```python
from build123d import *

# Parameters (mm, degrees)
F0_W     = 101.6
F0_H     = 9.525
F0_R     = 1.35255
F0_R_2   = 3.175
F1_DEPTH = 1.70942
F2_R     = 0.762
F3_SIZE  = 1.5875


with BuildPart() as f1:
    # F0 (on Top) → F1 (new body)
    with BuildSketch(Plane.XY):
        with Locations((-50.8, -4.7625)):
            Rectangle(F0_W, F0_H)
        with Locations((-97.63125, -3.96875)):
            Circle(F0_R, mode=Mode.SUBTRACT)
        with Locations((-65.057693, -3.96875)):
            Circle(F0_R, mode=Mode.SUBTRACT)
        with Locations((-50.8, -3.96875)):
            Circle(F0_R_2, mode=Mode.SUBTRACT)
        with Locations((-36.542307, -3.96875)):
            Circle(F0_R, mode=Mode.SUBTRACT)
        with Locations((-3.96875, -3.96875)):
            Circle(F0_R, mode=Mode.SUBTRACT)
    extrude(amount=F1_DEPTH)

    # F2
    f2_edges = [f1.edges().sort_by_distance(p)[0] for p in [
        (-101.6, 0, 0.85471),
        (0, 0, 0.85471),
    ]]
    fillet(f2_edges, radius=F2_R)

    # F3
    f3_edges = [f1.edges().sort_by_distance(p)[0] for p in [
        (0, -9.525, 0.85471),
        (-101.6, -9.525, 0.85471),
    ]]
    chamfer(f3_edges, length=F3_SIZE)


solid = f1.part
```
The listing builds one solid part. Answer for the finished solid, in the listing's coordinates (mm). Coordinates: 2 decimals unless noted, no trailing zeros. Loops run counter-clockwise (first coordinate to the right, second up) from the corner with the lowest first, then second, coordinate; pieces in that order, holes last. Notation, with made-up numbers: M -24,-21 L -1,-21 A7 ccw -1,-11 Z; hole C 63.25,50.25 d8. An arc over 180 degrees is marked long. Answer as CSV lines item,"result". Start each with the question number.
(1) Find the intervals of material crossed by L1, parallel to Y at x = -50.8, z = 1.3 (3 decimals); L2, parallel to X at y = -3.5, z = 0.5; L3, parallel to X at y = -3.25, z = 1.15, in increasing order. Write a range as [from, to].
(2) The part is cut by section A-A (x = -50.8). Give the vertices of the cut face in (y, z) (3 decimals), and give its area (3 significant figures).
(3) The part is cut by section B-B (z = 1.2). State how many separate pieces and enclosed holes the cut face has, and give its area (3 significant figures).
(4) The mould has two halves that part along X. Classify faces 1 (the flat face through (-101.6, -4, 1)), 2 (the flat face through (-51, -9.525, 1)), 3 (the cylindrical face through (-4.26, -5.29, 0.84)): pulls with the +X half, pulls with the -X half, needs draft (parallel to the pull), parting line crosses it, or undercut.
(5) Given pin 1 (2 mm diameter, centred on x = -97.63, y = -3.97, fed in from -Z), flat-ended and moving along its own axis, determine where the tip first touches the part or whether it passes through.
Determined:
1,L1,"[-9.525, -7.144], [-0.794, 0]"
1,L2,"[-101.6, -98.9], [-96.36, -66.33], [-63.79, -53.94], [-47.66, -37.81], [-35.27, -5.24], [-2.7, 0]"
1,L3,"[-101.6, -98.78], [-96.49, -66.2], [-63.91, -53.89], [-47.71, -37.69], [-35.4, -5.11], [-2.82, 0]"
2,outline,"M -9.525,0 L -7.144,0 L -7.144,1.709 L -9.525,1.709 Z; M -0.794,0 L 0,0 L 0,1.709 L -0.794,1.709 Z"
2,area,"5.43 mm2"
3,separate pieces,"1"
3,enclosed holes,"5"
3,area,"910 mm2"
4,face 1,"pulls with the -X half"
4,face 2,"needs draft"
4,face 3,"undercut"
5,pin 1,"through"
